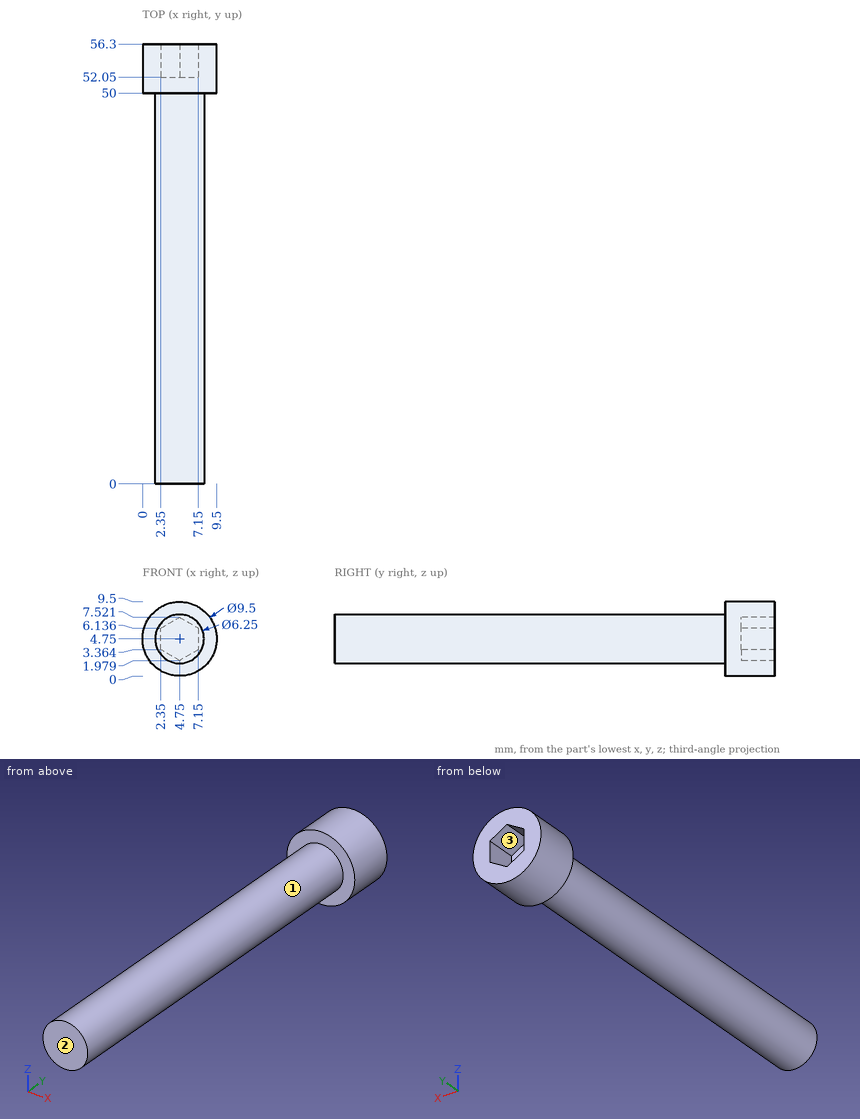
The drawing under review shows one solid part. Ordinate dimensions are in mm from its lowest x, y, z. Give positions to 0.01 mm unless a question says otherwise; leave off trailing zeros. Answer in a Markdown table with one row per item. Add a question column.
1. Insertion check: P1, Ø1, axis at x = 3, y = 17.5, coming from the +Z side; P2, Ø4, axis at x = 6, y = 6.5, coming from the +Z side (3 decimals); P3, Ø2, axis at x = 8, y = 37.5, coming from the +Z side. Each pin has a flat end and moves straight along its axis. Give the tip position at first contact, or say it passes through.
2. Wall thickness on line 1 along Z through (x, y) = (6.75, 14.5); line 2 along Y through (x, z) = (4.75, 9); line 3 along Y through (x, z) = (5.75, 5.5): over which ranges is each line inside the solid? List them lowest first. Write a range as [from, to].
3. Draft analysis for pull direction Z (two halves, no side actions). For the marked faces 1, 2 and 3, state which applies: +Z half, -Z half, draft (parallel to the pull), parting line (faces both ways), or undercut.
Ans:
| question | item | result |
|---|---|---|
| 1 | P1 | stops at z = 7.61 |
| 1 | P2 | stops at z = 7.875 |
| 1 | P3 | stops at z = 6.92 |
| 2 | line 1 | z = [2.35, 7.15] |
| 2 | line 2 | y = [50, 56.3] |
| 2 | line 3 | y = [0, 52.05] |
| 3 | face 1 | parting line |
| 3 | face 2 | draft |
| 3 | face 3 | undercut |
